from build123d import *

# Parameters (mm, degrees)
SKETCH_1_R                  = 4
EXTRUDE_1_DEPTH             = 39.1
EXTRUDE_2_DEPTH             = 39.1
HOLE_WIZARD_M32_D           = 3.15
PATTERN_LINEAR_2_COUNT      = 2
PATTERN_LINEAR_2_PITCH      = 34
PATTERN_LINEAR_2_COUNT_DIR2 = 2
PATTERN_LINEAR_2_PITCH_DIR2 = 34
SKETCH_10_W                 = 24
SKETCH_10_H                 = 12
CUT_EXTRUDE_2_DEPTH         = 2


with BuildPart() as part:
    # Эскиз1 → Бобышка-Вытянуть1 (new body)
    with BuildSketch(Plane(origin=(0, 0, 0), x_dir=(1, 0, 0), z_dir=(0, 1, 0))):
        with BuildLine():
            Line((-19.55, -10), (19.55, -10))
            Line((19.55, -10), (19.55, -6))
            Line((19.55, -6), (9.55, -6))
            Line((9.55, -6), (6, 0))
            ThreePointArc((6, 0), (0, 6), (-6, 0))
            Line((-6, 0), (-9.55, -6))
            Line((-9.55, -6), (-19.55, -6))
            Line((-19.55, -6), (-19.55, -10))
        make_face()
        Circle(SKETCH_1_R, mode=Mode.SUBTRACT)
    extrude(amount=EXTRUDE_1_DEPTH)

    # Эскиз5 → Бобышка-Вытянуть2 (add)
    with BuildSketch(Plane(origin=(19.55, 0, 0), x_dir=(0, 0, -1), z_dir=(1, 0, 0))):
        Polygon((-10, 0), (-15, 39.1), (-10, 39.1), align=None)
    extrude(amount=-EXTRUDE_2_DEPTH)

    # Сверло под метчик  спиральное M32 (through all)
    with Locations(Plane(origin=(0, -1.258197592, 9.839105167), x_dir=(1, 0, 0), z_dir=(0, -0.126844327, 0.991922636))):
        with Locations((-17, 3.818443269)):
            hole_wizard_m32 = Hole(HOLE_WIZARD_M32_D / 2)

    # Линейный массив2: Hole Wizard M32 2 × 2
    with Locations(*[Vector(1, 0, 0) * (i * PATTERN_LINEAR_2_PITCH) + Vector(0, 0.991922636, 0.126844327) * (j * PATTERN_LINEAR_2_PITCH_DIR2) for i in range(PATTERN_LINEAR_2_COUNT) for j in range(PATTERN_LINEAR_2_COUNT_DIR2) if (i, j) != (0, 0)]):
        add(hole_wizard_m32, mode=Mode.SUBTRACT)

    # Эскиз10 → Вырез-Вытянуть2 (cut)
    with BuildSketch(Plane(origin=(0, -1.258197592, 9.839105167), x_dir=(1, 0, 0), z_dir=(0, -0.126844327, 0.991922636))):
        with Locations((0, 5.268443269)):
            Rectangle(SKETCH_10_W, SKETCH_10_H)
    extrude(amount=-CUT_EXTRUDE_2_DEPTH, mode=Mode.SUBTRACT)


solid = part.part
Part model, mm, in its own coordinate system. A direction names the side the tool comes from. Give positions to 0.01 mm unless a question says otherwise; leave off trailing zeros. Loops run counter-clockwise (first coordinate to the right, second up) from the corner with the lowest first, then second, coordinate; pieces in that order, holes last. Notation, with made-up numbers: M -22,23 L -1,23 A29 cw -1,57 Z; hole C -17.5,85 d9. An arc over 180 degrees is marked long. Put each result on its own line as item: value. Start each with the question number.
1) Saw through at B-B (z = -3.5). List the corners of the cut face in (x, y).
2) Pull direction X, two halves, no side cores. Call faces 6 (the cylindrical face through (16.15, 4.14, 8.18)), 7 (the flat face through (19.55, 24, 9)), 8 (the cylindrical face through (0, 19, -6)), 9 (the flat face through (-19.55, 24, 9)): +X half, -X half, draft (parallel to the pull), parting line (faces both ways), or undercut.
3) 3-axis set-ups, long thin cutter, end or side, ignore diameter. For faces 1 (the flat face through (0.27, 23.62, 13.02)), 2 (the flat face through (0, 39.1, 9)), 3 (the flat face through (15, 19, 6)), 4 (the flat face through (-14, 19, 6)), 5 (the flat face through (-0.168, 10.044, 10.29)): which of +Z, -Z, +X, -X, +Y, -Y reach the whole face in a straight line?
4) Probe probe 1 along X at (y, z) = (3.5, 1.75); probe 2 along Z at (x, y) = (0, 20); probe 3 along Z at (x, y) = (0, 16). List the from-to ranges inside material, lowest first.
5) Saw through at A-A (x = 0). List the corners of the cut face in (y, z).
6) Saw through at C-C (y = 4). State how many separate pieces and enclosed holes the cut face has, then the cut area to 3 significant figures.
7) Saw through at D-D (y = 32.5). List the corners of the cut face in (x, z), then the cut area to 3 significant figures.
8) Flat gauge pins, fed straight in: pin 1 (4 mm diameter, centred on x = -15.5, y = 19.5, fed in from -Z); pin 2 (6 mm diameter, centred on x = 12.5, y = 8, fed in from +Z); pin 3 (8 mm diameter, centred on x = -12, y = 26.5, fed in from -Z). Where does each tip first touch, or does it go through?
Numbers:
1. outline: M -4.87,0 L -1.94,0 L -1.94,39.1 L -4.87,39.1 Z; M 1.94,0 L 4.87,0 L 4.87,39.1 L 1.94,39.1 Z
2. face 6: undercut
2. face 7: +X half
2. face 8: parting line
2. face 9: -X half
3. face 1: +Z, +X, -X, -Y
3. face 2: +Z, -Z, +X, -X, +Y
3. face 3: -Z, +X, +Y, -Y
3. face 4: -Z, -X, +Y, -Y
3. face 5: -Y
4. probe 1: -7.04 to -3.6, 3.6 to 7.04
4. probe 2: -6 to -4, 4 to 12.56
4. probe 3: -6 to -4, 4 to 12.05
5. outline: M 0,-6 L 39.1,-6 L 39.1,-4 L 0,-4 Z; M 0,4 L 39.1,4 L 39.1,15 L 9.92,11.27 L 10.17,9.28 L 0,7.98 Z
6. separate pieces: 3
6. enclosed holes: 1
6. area: 210 mm^2
7. outline: M -19.55,6 L -9.55,6 L -6,0 A6 ccw 6,0 L 9.55,6 L 19.55,6 L 19.55,14.16 L -19.55,14.16 Z; hole C 0,0 d8
7. area: 418 mm^2
8. pin 1: z = 6
8. pin 2: z = 11.41
8. pin 3: z = 3.38
